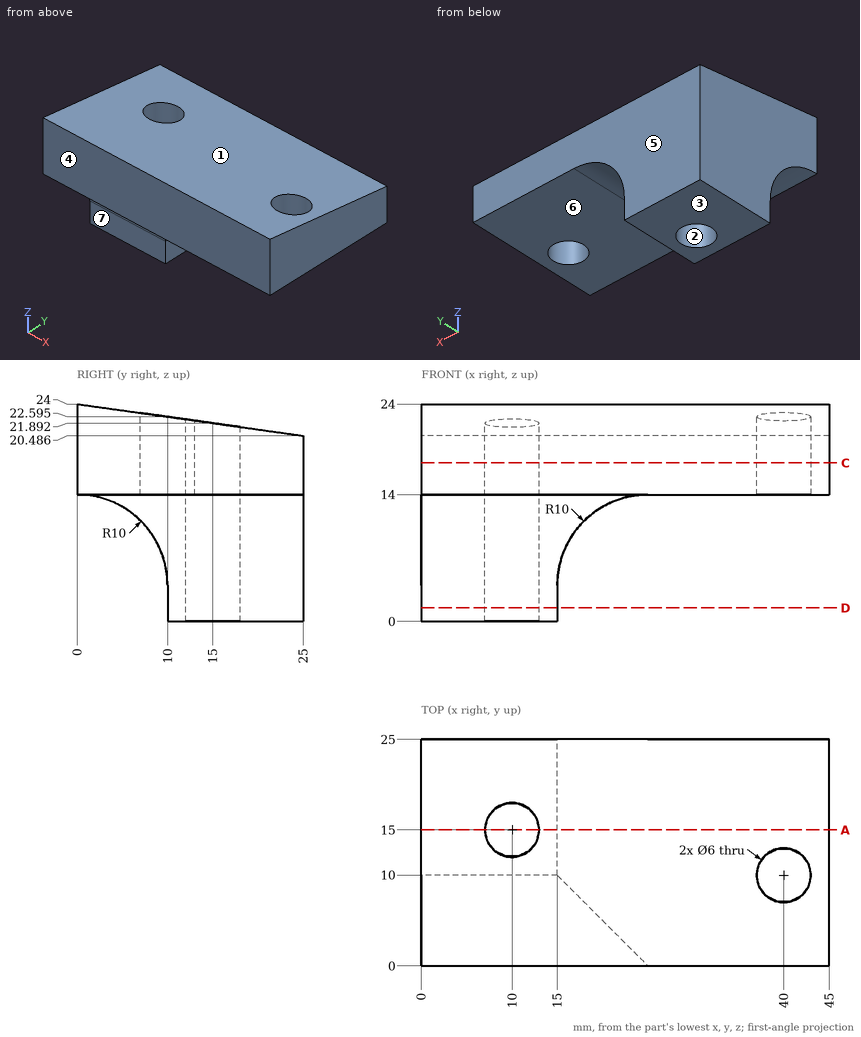
Part print with two shaded views. Sizes in mm from the minimum x, y, z corner. A direction names the side the tool comes from. Round coordinates to 2 decimals unless told otherwise and drop trailing zeros. Write each loop counter-clockwise with the first axis right and the second up, starting at its lowest first coordinate (ties: lowest second). Pieces come first, ordered by that corner, then holes. Notation, with made-up numbers: (76.5, -27.5) - (110.5, -27.5) arc R21 ccw to (110.5, -5.5) - close; hole circle Ø8 at (6.25, 87.5). An arc over 180 degrees is marked (long way). Answer as CSV lines item,"result".
Q1. Pull direction Y, two halves, no side cores. Call the marked faces 1, 2, 3 and 4: +Y half, -Y half, draft (parallel to the pull), parting line (faces both ways), or undercut.
Report:
face 1,"+Y half"
face 2,"undercut"
face 3,"draft"
face 4,"-Y half"
Q2. Cut at D-D (z = 1.5). Write the cut outline in (x, y), and give its area (3 significant figures).
Report:
outline,"(0, 10) - (15, 10) - (15, 25) - (0, 25) - close; hole circle Ø6 at (10, 15)"
area,"197 mm^2"
Q3. Tool access for the marked faces 5, 6 and 7: list every direction of +Z, -Z, +X, -X, +Y, -Y with a clear straight run to the whole face (end or side of a thin tool).
Report:
face 5,"+Z, -Z, +X, -X, +Y"
face 6,"-Z, +X, +Y, -Y"
face 7,"-Z, +X, -X, -Y"
Q4. Drill centre lines: probe 1 along X at (y, z) = (10, 18.5); probe 2 along Y at (x, z) = (40, 15.5); probe 3 along Y at (x, z) = (4, 3.75). Where is each one in solid material? Low to high. Write a range as [from, to].
Report:
probe 1,"x = [0, 37], [43, 45]"
probe 2,"y = [0, 7], [13, 25]"
probe 3,"y = [10, 25]"
Q5. Drop flat-ended pins along their axis: pin 1 (2 mm diameter, centred on y = 8.5, z = 12, fed in from -X); pin 2 (5 mm diameter, centred on x = 10, y = 15, fed in from -Z); pin 3 (12 mm diameter, centred on x = 37.5, y = 16, fed in from +Z); pin 4 (7 mm diameter, centred on x = 40, y = 10, fed in from -Z). Give the stop position or say it passes through.
Report:
pin 1,"stops at x = 0"
pin 2,"passes through"
pin 3,"stops at z = 22.59"
pin 4,"stops at z = 14"
Q6. Cut at C-C (z = 17.5). Write the cut outline in (x, y), and give its area (3 significant figures).
Report:
outline,"(0, 0) - (45, 0) - (45, 25) - (0, 25) - close; hole circle Ø6 at (10, 15); hole circle Ø6 at (40, 10)"
area,"1,070 mm^2"
Q7. Cut at A-A (y = 15). Write the cut outline in (x, z).
Report:
outline,"(0, 0) - (7, 0) - (7, 21.89) - (0, 21.89) - close; (13, 0) - (15, 0) - (15, 4) arc R10 cw to (25, 14) - (45, 14) - (45, 21.89) - (13, 21.89) - close"
